Input: dimensioned drawing with shaded views. Units: mm. Origin: part minimum x, y, z. A direction names the side the tool comes from. Round coordinates to 2 decimals unless told otherwise and drop trailing zeros. Loops run counter-clockwise (first coordinate to the right, second up) from the corner with the lowest first, then second, coordinate; pieces in that order, holes last. Notation, with made-up numbers: M 84,57 L 106,57 A27 ccw 106,86 Z; hole C 70.5,29 d3. An arc over 180 degrees is marked long. Use one line per item in the form item = value. Start each with the question number.
Q1. Ray query, line 1 along Y through (x, z) = (15, 19.4); line 2 along Z through (x, y) = (52.5, 61); line 3 along X through (y, z) = (23.5, 8). Return the intervals inside material, ascending.
Q2. First-contact query: P1, Ø2.5, axis at x = 53, z = 20, coming from the -Y side; P2, Ø6, axis at x = 30, z = 25.5, coming from the -Y side; P3, Ø2, axis at x = 8.5, z = 18, coming from the -Y side; P4, Ø3.5, axis at y = 67, z = 4, coming from the +X side. Flat tips, straight axial feed; report the tip coordinate or a pass-through.
Q3. Section query B-B, the plane y = 51. Output: boundary loops of the cut face in (x, z), and give its area (3 significant figures).
Q4. Section query A-A, the plane x = 15. Output: boundary loops of the cut face in (y, z).
Q5. Access query for the marked faces 1, 2 and 3. Directions: +Z, -Z, +X, -X, +Y, -Y. A direction counts if a zero-diameter tool reaches every point of the face in a straight line with its end or side. Return the directions, or none.
Q6. Section query D-D, the plane z = 20. Output: boundary loops of the cut face in (x, y), and give its area (3 significant figures).
Q7. Section query C-C, the plane y = 75. Output: boundary loops of the cut face in (x, z).
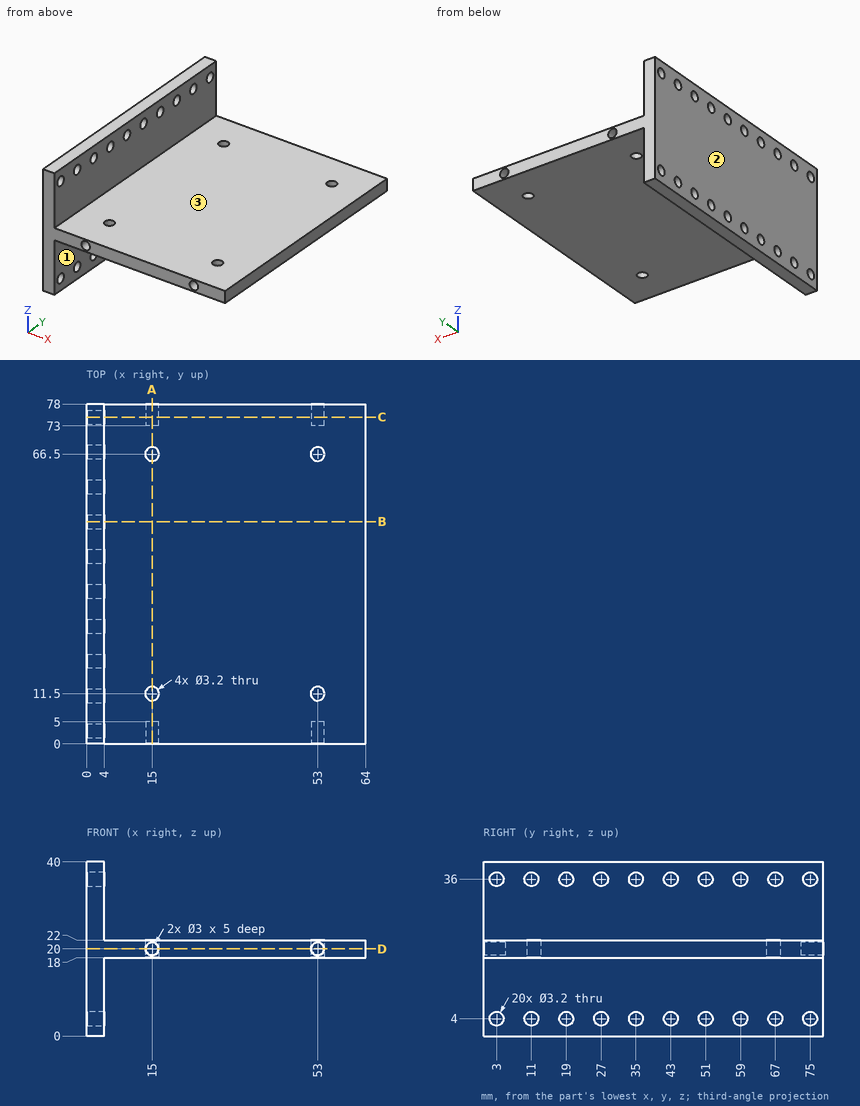
Results found:
q1.line_1 = 5 to 9.9, 13.1 to 64.9, 68.1 to 73
q1.line_2 = 18 to 22
q1.line_3 = 0 to 4
q2.P1 = 5
q2.P2 = through
q2.P3 = 0
q2.P4 = 4
q3.outline = M 0,0 L 4,0 L 4,2.4 L 0,2.4 Z; M 0,5.6 L 4,5.6 L 4,18 L 64,18 L 64,22 L 4,22 L 4,34.4 L 0,34.4 Z; M 0,37.6 L 4,37.6 L 4,40 L 0,40 Z
q3.area = 374 mm²
q4.outline = M 0,18 L 9.9,18 L 9.9,22 L 0,22 L 0,21.5 L 5,21.5 L 5,18.5 L 0,18.5 Z; M 13.1,18 L 64.9,18 L 64.9,22 L 13.1,22 Z; M 68.1,18 L 78,18 L 78,18.5 L 73,18.5 L 73,21.5 L 78,21.5 L 78,22 L 68.1,22 Z
q5.face_1 = -Z, +X, +Y, -Y
q5.face_2 = +Z, -Z, -X, +Y, -Y
q5.face_3 = +Z, +X, +Y, -Y
q6.outline = M 0,0 L 13.5,0 L 13.5,5 L 16.5,5 L 16.5,0 L 51.5,0 L 51.5,5 L 54.5,5 L 54.5,0 L 64,0 L 64,78 L 54.5,78 L 54.5,73 L 51.5,73 L 51.5,78 L 16.5,78 L 16.5,73 L 13.5,73 L 13.5,78 L 0,78 Z; hole C 15,11.5 d3.2; hole C 15,66.5 d3.2; hole C 53,11.5 d3.2; hole C 53,66.5 d3.2
q6.area = 4,900 mm²
q7.outline = M 0,0 L 4,0 L 4,2.4 L 0,2.4 Z; M 0,5.6 L 4,5.6 L 4,18 L 64,18 L 64,22 L 4,22 L 4,34.4 L 0,34.4 Z; M 0,37.6 L 4,37.6 L 4,40 L 0,40 Z; hole C 15,20 d3; hole C 53,20 d3
